Verification items for the finished model (mm, model axes). Give positions to 0.01 mm unless a question says otherwise; leave off trailing zeros. Order: outer loops, then holes, each group sorted by start corner. A loop starts at its lowest first (then second) coordinate and runs counter-clockwise, first axis right, second up.
Autodesk Inventor part; units mm, degrees
ref_plane "YZ Plane" through (0, 0, 0) normal (1, 0, 0) x (0, 1, 0)
ref_plane "XZ Plane" through (0, 0, 0) normal (0, 1, 0) x (-1, 0, 0)
ref_plane "XY Plane" through (0, 0, 0) normal (0, 0, 1) x (1, 0, 0)
sketch "スケッチ1" plane through (0, 0, 0) normal (0, 0, 1) x (1, 0, 0)
  circle A0 centre (0, 0) radius 3
  circle A1 centre (0, 0) radius 1.5
  dimension "d0" = 6
  dimension "d1" = 3
extrude "押し出し1" add sketch "スケッチ1" along normal blind 4.5
chamfer "面取り1" distance 2 distance2 1 1 edges at (-3, 0, 0) measured on face at (2.9903, -0.2414, 3)
sketch "スケッチ6" plane through (0, 0, 4.5) normal (0, 0, 1) x (1, 0, 0)
  circle A0 centre (0, 0) radius 2.05
  dimension "d23" = 4.1
extrude "押し出し4" cut sketch "スケッチ6" against normal blind 2
properties part number "Magnet_Simple"
(1) Section check A-A, the plane y = 0. Enter the section's corners in (x, z), then the cut area to 3 significant figures.
Solved:
outline: (-3, 2) - (-2, 0) - (-1.5, 0) - (-1.5, 2.5) - (-2.05, 2.5) - (-2.05, 4.5) - (-3, 4.5) - close; (1.5, 0) - (2, 0) - (3, 2) - (3, 4.5) - (2.05, 4.5) - (2.05, 2.5) - (1.5, 2.5) - close
area: 9.30 mm2
(2) Go/stop test with flat-tipped pins: pin 1 (1.5 mm diameter, centred on y = 2, z = 4, fed in from -X); pin 2 (1.5 mm diameter, centred on x = -0.5, y = 2, fed in from -Z). Record where each tip stops, or that it passes through.
Solved:
pin 1: stops at x = -2.73
pin 2: stops at z = 0
(3) Release check for a two-part mould opening along Y. For faces 1 (the flat face through (2, -1, 4.5)), 2 (the cylindrical face through (-3, 0, 3)), 3 (the cylindrical face through (-1.5, -0.07, 1.23)) record: pulls with the +Y half, pulls with the -Y half, needs draft (parallel to the pull), parting line crosses it, or undercut.
Solved:
face 1: needs draft
face 2: parting line crosses it
face 3: undercut
(4) Section check D-D, the plane z = 2.3. Enter the section's corners in (x, y).
Solved:
outline: circle Ø6 at (0, 0); hole circle Ø3 at (0, 0)
(5) Section check C-C, the plane z = 3.4. Enter the section's corners in (x, y).
Solved:
outline: circle Ø6 at (0, 0); hole circle Ø4.1 at (0, 0)
(6) Scan lines: line 1 (Y direction, x = 0, z = 3.75); line 2 (Z direction, x = 1.5, y = -1.25); line 3 (Y direction, x = 0, z = 1.2). Record each from-to range of solid material in increasing order.
Solved:
line 1: y = -3 to -2.05, 2.05 to 3
line 2: z = 0 to 2.5
line 3: y = -2.6 to -1.5, 1.5 to 2.6
